from build123d import *

# Parameters (mm, degrees)
SKETCH1_R           = 46
SKETCH1_R_2         = 3.5
BOSS_EXTRUDE1_DEPTH = 20
FILLET1_R           = 1
SKETCH2_R           = 12
BOSS_EXTRUDE2_DEPTH = 10
SKETCH3_R           = 33
CUT_EXTRUDE1_DEPTH  = 14
SKETCH4_R           = 2.5
CUT_EXTRUDE2_DEPTH  = 6
SKETCH5_R           = 7
CUT_EXTRUDE3_DEPTH  = 10
CHAMFER1_SIZE       = 1
CHAMFER1_SIZE2      = 1.732050808
SKETCH6_R           = 4
CUT_EXTRUDE4_DEPTH  = 80


with BuildPart() as part:
    # Sketch1 → Boss-Extrude1 (new body)
    with BuildSketch(Plane(origin=(0, 0, 0), x_dir=(1, 0, 0), z_dir=(0, 1, 0))):
        with Locations(Location((0, 0, 0), (0, 0, 270))):
            Circle(SKETCH1_R)
        with Locations(Location((0, 36, 0), (0, 0, 270))):
            Circle(SKETCH1_R_2, mode=Mode.SUBTRACT)
        with Locations(Location((31.176914536, 18, 0), (0, 0, 270))):
            Circle(SKETCH1_R_2, mode=Mode.SUBTRACT)
        with Locations(Location((31.176914536, -18, 0), (0, 0, 270))):
            Circle(SKETCH1_R_2, mode=Mode.SUBTRACT)
        with Locations(Location((0, -36, 0), (0, 0, 270))):
            Circle(SKETCH1_R_2, mode=Mode.SUBTRACT)
        with Locations(Location((-31.176914536, -18, 0), (0, 0, 270))):
            Circle(SKETCH1_R_2, mode=Mode.SUBTRACT)
        with Locations(Location((-31.176914536, 18, 0), (0, 0, 270))):
            Circle(SKETCH1_R_2, mode=Mode.SUBTRACT)
    extrude(amount=BOSS_EXTRUDE1_DEPTH)

    # Fillet1
    fillet1_edges = [part.edges().sort_by_distance(p)[0] for p in [
        (0, 20, -46),
    ]]
    fillet(fillet1_edges, radius=FILLET1_R)

    # Sketch2 → Boss-Extrude2 (add)
    with BuildSketch(Plane(origin=(0, 20, 0), x_dir=(1, 0, 0), z_dir=(0, 1, 0))):
        with Locations(Location((0, 0, 0), (0, 0, 270))):
            Circle(SKETCH2_R)
    extrude(amount=BOSS_EXTRUDE2_DEPTH)

    # Sketch3 → Cut-Extrude1 (cut)
    with BuildSketch(Plane.XZ):
        Circle(SKETCH3_R)
    extrude(amount=-CUT_EXTRUDE1_DEPTH, mode=Mode.SUBTRACT)

    # Sketch4 → Cut-Extrude2 (cut)
    with BuildSketch(Plane.XZ.offset(-14)):
        with Locations(Location((0, 0, 0), (0, 0, 270))):
            Circle(SKETCH4_R)
    extrude(amount=-CUT_EXTRUDE2_DEPTH, mode=Mode.SUBTRACT)

    # Sketch5 → Cut-Extrude3 (cut)
    with BuildSketch(Plane(origin=(0, 30, 0), x_dir=(1, 0, 0), z_dir=(0, 1, 0))):
        with Locations(Location((0, 0, 0), (0, 0, 270))):
            Circle(SKETCH5_R)
    extrude(amount=-CUT_EXTRUDE3_DEPTH, mode=Mode.SUBTRACT)

    # Chamfer1
    chamfer1_edges = [part.edges().sort_by_distance(p)[0] for p in [
        (0, 30, -7),
    ]]
    chamfer1_side = [part.faces().sort_by_distance(p)[0] for p in [
        (0, 30, -11.660588745),
    ]]
    chamfer(chamfer1_edges, length=CHAMFER1_SIZE, length2=CHAMFER1_SIZE2, reference=chamfer1_side[0])

    # Sketch6 → Cut-Extrude4 (cut)
    with BuildSketch(Plane(origin=(0, 0, 0), x_dir=(0, 0, -1), z_dir=(1, 0, 0))):
        with Locations(Location((0, 8, 0), (0, 0, 180))):
            Circle(SKETCH6_R)
    extrude(amount=CUT_EXTRUDE4_DEPTH, mode=Mode.SUBTRACT)


solid = part.part
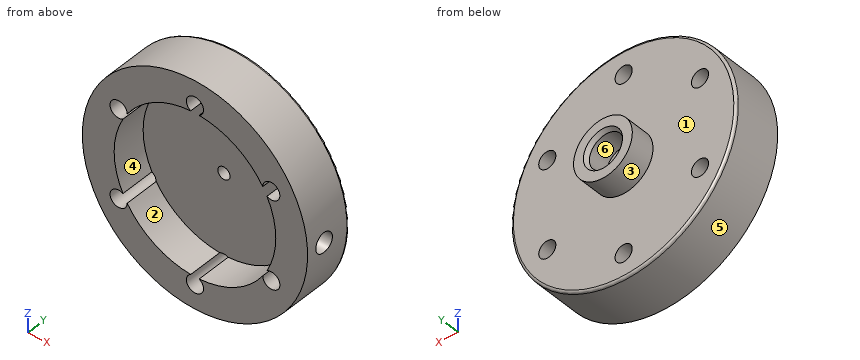
Work out the finished part from the listing and answer in its coordinate system (mm). Face numbers are marked on the shaded views. A direction names the side the tool comes from. Round coordinates to 2 decimals unless told otherwise and drop trailing zeros. Write each loop counter-clockwise with the first axis right and the second up, starting at its lowest first coordinate (ties: lowest second). Pieces come first, ordered by that corner, then holes. Notation, with made-up numbers: M 63,-26.75 L 85,-26.75 A27 cw 85,-0.75 Z; hole C 9.25,-33.75 d3. An arc over 180 degrees is marked long. Use a Markdown table: item, result.
1) Flat-ended cylindrical pins translate along their axes: pin 1 (10 mm diameter, centred on y = 12.5, z = 13.5, fed in from -X); pin 2 (2 mm diameter, centred on y = 22, z = -8.5, fed in from -X); pin 3 (9 mm diameter, centred on x = -31.18, z = 18, fed in from -Y); pin 4 (12 mm diameter, centred on y = 16.5, z = 28.5, fed in from -X). Find the tip coordinate at first contact, or state that the pin passes through.
Taken from the geometry:
| item | result |
|---|---|
| pin 1 | stops at x = -45.21 |
| pin 2 | stops at x = -9.37 |
| pin 3 | stops at y = 0 |
| pin 4 | stops at x = -40.12 |
2) The part is cut by section B-B on y = 10. Give the vertices of the cut face in (x, z).
Taken from the geometry:
| item | result |
|---|---|
| outline | M -29.4,-14.98 A33 cw -29.4,14.98 A3.5 cw long -27.68,17.97 A33 cw -1.73,32.95 A3.5 cw long 1.73,32.95 A33 cw 27.68,17.97 A3.5 cw long 29.4,14.98 A33 cw 32.82,3.46 L 45.87,3.46 A46 ccw long 45.87,-3.46 L 32.82,-3.46 A33 cw 29.4,-14.98 A3.5 cw long 27.68,-17.97 A33 cw 1.73,-32.95 A3.5 cw long -1.73,-32.95 A33 cw -27.68,-17.97 A3.5 cw long Z |
3) The part is cut by section A-A on y = 17. Give the vertices of the cut face in (x, z), plus the area to 3 significant figures.
Taken from the geometry:
| item | result |
|---|---|
| outline | C 0,0 d92; hole C -31.18,-18 d7; hole C -31.18,18 d7; hole C 0,-36 d7; hole C 0,36 d7; hole C 0,0 d5; hole C 31.18,-18 d7; hole C 31.18,18 d7 |
| area | 6,400 mm2 |
4) Which of the six approach directions +Z, -Z, +X, -X, +Y, -Y give full straight-line access (tool end or side, diameter ignored) to the marked faces 4, 5 and 6?
Taken from the geometry:
| item | result |
|---|---|
| face 4 | -Y |
| face 5 | +Y, -Y |
| face 6 | +Y |
5) Determine the mould class of the marked faces 1, 2 and 3 for opening direction Z: pulls with the +Z half, pulls with the -Z half, needs draft (parallel to the pull), parting line crosses it, or undercut.
Taken from the geometry:
| item | result |
|---|---|
| face 1 | needs draft |
| face 2 | undercut |
| face 3 | parting line crosses it |
6) Consider line 1 (Y direction, x = -42, z = -2); line 2 (Z direction, x = -25, y = 13); line 3 (Z direction, x = -3.5, y = 21). Determine where each line is inside the solid, lowest interval first. Write a range as [from, to].
Taken from the geometry:
| item | result |
|---|---|
| line 1 | y = [0, 20] |
| line 2 | z = [-38.61, -21.54], [21.54, 38.61] |
| line 3 | z = [-11.48, -6.06], [6.06, 11.48] |
